The listing builds one solid part. Answer for the finished solid, in the listing's coordinates (mm). A direction names the side the tool comes from. Round coordinates to 2 decimals unless told otherwise and drop trailing zeros. Loops run counter-clockwise (first coordinate to the right, second up) from the corner with the lowest first, then second, coordinate; pieces in that order, holes last. Notation, with made-up numbers: (74.5, -25) -> (89.5, -25) arc R23 ccw to (89.5, 2) -> close; hole circle Ø7 at (22.25, 14). An arc over 180 degrees is marked (long way). Write each question's results on one line, items separated by ' | '. Start each with the question number.
from build123d import *

# Parameters (mm, degrees)
TABAN_FLAN_1_DEPTH = 50


# Sheet-metal steps are written as plain solids
with BuildPart() as part:
    # Çizim1 → Taban-Flanş1 (new body)
    with BuildSketch(Plane.XY):
        with BuildLine():
            Line((0, 0), (218.5, 0))
            ThreePointArc((218.5, 0), (276, 50), (333.5, 0))
            Line((333.5, 0), (360, 0))
            Line((360, 0), (449, 0))
            Line((449, 0), (458.997671741, 0.215777088))
            Line((458.997671741, 0.215777088), (455.997671741, 139.215777088))
            ThreePointArc((455.997671741, 139.215777088), (447.698955646, 153.213358252), (432.909011054, 160))
            Line((432.909011054, 160), (367.081412811, 160))
            ThreePointArc((367.081412811, 160), (323.554697394, 218.317011668), (374.513743955, 270.265297284))
            Line((374.513743955, 270.265297284), (434.798113421, 270.265297284))
            Line((434.798113421, 270.265297284), (444.798113421, 270.265297284))
            Line((444.798113421, 270.265297284), (444.798113421, 315.516988045))
            ThreePointArc((444.798113421, 315.516988045), (432.826102146, 329.550683033), (418.309236409, 340.931994828))
            Line((418.309236409, 340.931994828), (348.808103312, 358.867771111))
            ThreePointArc((348.808103312, 358.867771111), (316.270646866, 355.31487857), (287.772711056, 339.215910531))
            Line((287.772711056, 339.215910531), (171.828858079, 213.879290682))
            ThreePointArc((171.828858079, 213.879290682), (144.61514494, 194.164293468), (113.814091907, 180.726941422))
            ThreePointArc((113.814091907, 180.726941422), (82.931673061, 178.777598724), (53.149679292, 187.177395023))
            Line((53.149679292, 187.177395023), (53.149679292, 80.862415296))
            Line((53.149679292, 80.862415296), (0, 0))
        make_face()
    extrude(amount=TABAN_FLAN_1_DEPTH)


solid = part.part
Item 1: Each of these flat-tipped pins is pushed along its axis until it touches: pin 1 Ø6 at (x, y) = (303, 101.5) entering from -Z; pin 2 Ø1 at (y, z) = (166.5, 23) entering from +X; pin 3 Ø25 at (x, z) = (389.5, 22.5) entering from +Y; pin 4 Ø3 at (y, z) = (100, 19.5) entering from +X. Where does it stop, or does it pass through?
Item 2: Determine the mould class of faces 1 (the flat face through (384.045, 349.774, 24.65)), 2 (the cylindrical face through (83.365, 178.733, 24.65)), 3 (the flat face through (108, 0, 25)) for opening direction X: +X half, -X half, draft (parallel to the pull), parting line (faces both ways), or undercut.
Item 3: Straight lines are drawn through the part: L1, parallel to X at y = 38.5, z = 32; L2, parallel to X at y = 22.5, z = 35; L3, parallel to Y at x = 337, z = 29. For each, find the intervals that lie inside material, in ascending order. Write a range as [from, to].
Item 4: For faces 4 (the flat face through (409, 270.265, 25)), 5 (the flat face through (53.15, 135, 25)), 6 (the flat face through (444.798, 293, 25)), 7 (the cylindrical face through (145.024, 194.399, 24.65)), determine the directions among +Z, -Z, +X, -X, +Y, -Y from which every point of the face is accessible in a straight line to the end or side of a thin tool.
Item 5: The part is cut by section A-A, the plane x = 424. Give the vertices of the cut face in (y, z).
Item 6: The part is cut by section D-D, the plane x = 262.5. Give the vertices of the cut face in (y, z), plus the area to 3 significant figures.
Item 7: The part is cut by section C-C, the plane y = 281.5. Give the vertices of the cut face in (x, z).
Item 8: The part is cut by section B-B, the plane z = 8. Give the vertices of the cut face in (x, y) (1 decimal), plus the area to 3 significant figures.
Report:
1) pin 1: stops at z = 0 | pin 2: stops at x = 351.61 | pin 3: stops at y = 351.59 | pin 4: stops at x = 456.88
2) face 1: +X half | face 2: undercut | face 3: draft
3) L1: x = [25.31, 241.31], [310.69, 458.17] | L2: x = [14.79, 226.63], [325.37, 458.52] | L3: y = [0, 178.04], [251.08, 359.12]
4) face 4: +Z, -Z, +X | face 5: +Z, -Z, -X, +Y | face 6: +Z, -Z, +X, +Y | face 7: +Z, -Z, +Y
5) outline: (0, 0) -> (160, 0) -> (160, 50) -> (0, 50) -> close; (270.27, 0) -> (337.02, 0) -> (337.02, 50) -> (270.27, 50) -> close
6) outline: (48.41, 0) -> (311.9, 0) -> (311.9, 50) -> (48.41, 50) -> close | area: 13,200 mm2
7) outline: (234.38, 0) -> (444.8, 0) -> (444.8, 50) -> (234.38, 50) -> close
8) outline: (0, 0) -> (218.5, 0) arc R58.1 cw to (333.5, 0) -> (449, 0) -> (459, 0.2) -> (456, 139.2) arc R27.3 ccw to (432.9, 160) -> (367.1, 160) arc R55.9 cw to (374.5, 270.3) -> (444.8, 270.3) -> (444.8, 315.5) arc R92.6 ccw to (418.3, 340.9) -> (348.8, 358.9) arc R81.3 ccw to (287.8, 339.2) -> (171.8, 213.9) arc R156.2 cw to (113.8, 180.7) arc R92 cw to (53.1, 187.2) -> (53.1, 80.9) -> close | area: 96,500 mm2
